```python
from build123d import *

# Parameters (mm, degrees)
EXTRUDE_1_DEPTH     = 4
SKETCH_3_R          = 9
EXTRUDE_2_DEPTH     = 7
SKETCH_4_R          = 3
CUT_EXTRUDE_1_DEPTH = 49.751330175
SKETCH_5_R          = 6
CUT_EXTRUDE_2_DEPTH = 10
SKETCH_7_R          = 5.5
CUT_EXTRUDE_3_DEPTH = 50.484262082
HOLE_WIZARD_M4_1_D  = 3.3
SCALE1_SCALE        = 2


with BuildPart() as part:
    # 草图1 → 凸台-拉伸1 (new body)
    with BuildSketch(Plane(origin=(0, 0, 0), x_dir=(1, 0, 0), z_dir=(0, 1, 0))):
        with BuildLine():
            Line((-8.109776452, 3.902758754), (-25.406517635, -32.039176982))
            ThreePointArc((-25.406517635, -32.039176982), (-23, -39.837168574), (-15.043482365, -38.022278184))
            Line((-15.043482365, -38.022278184), (0.302963304, -15.526261061))
            Line((0.302963304, -15.526261061), (7.351564548, -25.039059461))
            ThreePointArc((7.351564548, -25.039059461), (12.25592959, -26.282925824), (14.455537758, -21.72642235))
            Line((14.455537758, -21.72642235), (8.752682732, 2.095362733))
            ThreePointArc((8.752682732, 2.095362733), (0.95916746, 8.948742805), (-8.109776452, 3.902758754))
        make_face()
    extrude(amount=EXTRUDE_1_DEPTH)

    # 草图3 → 凸台-拉伸2 (add)
    with BuildSketch(Plane(origin=(0, 4, 0), x_dir=(1, 0, 0), z_dir=(0, 1, 0))):
        with Locations(Location((0, 0, 0), (0, 0, 154.301222305))):
            Circle(SKETCH_3_R)
    extrude(amount=EXTRUDE_2_DEPTH)

    # 草图4 → 切除-拉伸1 (cut, through all)
    with BuildSketch(Plane(origin=(0, 4, 0), x_dir=(1, 0, 0), z_dir=(0, 1, 0))):
        with Locations(Location((-20, -34.641016151, 0), (0, 0, 270))):
            Circle(SKETCH_4_R)
    extrude(amount=-CUT_EXTRUDE_1_DEPTH, mode=Mode.SUBTRACT)

    # 草图5 → 切除-拉伸2 (cut)
    with BuildSketch(Plane.XZ):
        with Locations(Location((0, 0, 0), (0, 0, 270))):
            Circle(SKETCH_5_R)
    extrude(amount=-CUT_EXTRUDE_2_DEPTH, mode=Mode.SUBTRACT)

    # 草图7 → 切除-拉伸3 (cut, through all)
    with BuildSketch(Plane(origin=(0, 11, 0), x_dir=(1, 0, 0), z_dir=(0, 1, 0))):
        with Locations(Location((0, 0, 0), (0, 0, 270))):
            Circle(SKETCH_7_R)
    extrude(amount=-CUT_EXTRUDE_3_DEPTH, mode=Mode.SUBTRACT)

    # M4 螺纹孔1 (through all)
    with Locations(Plane(origin=(0, 4, 0), x_dir=(1, 0, 0), z_dir=(0, 1, 0))):
        with Locations((10.565456544, -22.657694676)):
            Hole(HOLE_WIZARD_M4_1_D / 2)


with BuildPart() as part_1:
    # Scale1: scaled about (-4.168101576, 3.295275318, 12.285042226)
    add(part.part.scale(SCALE1_SCALE).moved(Location((4.168101576, -3.295275318, -12.285042226))))


solid = part_1.part
```
Design review of the part built by this model. Coordinates are the model's own, in mm. A direction names the side the tool comes from. Coordinates: 2 decimals unless noted, no trailing zeros. Order: outer loops, then holes, each group sorted by start corner. A loop starts at its lowest first (then second) coordinate and runs counter-clockwise, first axis right, second up. Notation, with made-up numbers: (68, -25) - (73, -25) arc R27 ccw to (73, 10) - close; hole circle Ø1 at (31, -23). An arc over 180 degrees is marked (long way). Answer in a Markdown table with one row per item.
(1) Clearance check with flat-ended pins moving along their axes: pin 1 (3 mm diameter, centred on y = 7, z = -1.5, fed in from -X); pin 2 (10.5 mm diameter, centred on x = 25.3, z = 33.03, fed in from +Y); pin 3 (2 mm diameter, centred on x = -1, y = 7, fed in from +Z). State where each tip first meets the part, or that it passes through.
Checked values:
| item | result |
|---|---|
| pin 1 | x = -11.25 |
| pin 2 | y = 4.7 |
| pin 3 | z = 5.23 |
(2) Consider section D-D on x = -39. State the section outline as (y, z) points.
Checked values:
| item | result |
|---|---|
| outline | (-3.3, 35.91) - (4.7, 35.91) - (4.7, 51.9) - (-3.3, 51.9) - close; (-3.3, 62.09) - (4.7, 62.09) - (4.7, 68.57) - (-3.3, 68.57) - close |
(3) Consider section B-B on y = 0. State the section outline as (x, z) points, plus the area to 3 significant figures.
Checked values:
| item | result |
|---|---|
| outline | (-46.64, 51.79) - (-12.05, -20.09) arc R18 ccw to (21.67, -16.48) - (33.08, 31.17) arc R8 ccw to (18.87, 37.79) - (4.77, 18.77) - (-25.92, 63.76) arc R12 ccw to start; hole circle Ø12 at (-35.83, 57); hole circle Ø24 at (4.17, -12.29); hole circle Ø6.6 at (25.3, 33.03) |
| area | 3,310 mm^2 |
(4) For faces 4 (the flat face through (-6, 16.705, -18)), 5 (the flat face through (-8, -3.295, 19)), 6 (the flat face through (-10.8, 0.6, 41.6)), list the 3-axis set-ups (+Z, -Z, +X, -X, +Y, -Y) from which the entire face can be reached by the end or side of a thin tool; tool diameter is ignored.
Checked values:
| item | result |
|---|---|
| face 4 | -Y |
| face 5 | +Z, -Z, +X, -X, -Y |
| face 6 | +Z, +Y, -Y |
(5) The part is to be moulded in two halves that separate along Z. For faces 1 (the flat face through (15, 18.705, -16)), 2 (the cylindrical face through (27.918, 0.649, 35.038)), 3 (the flat face through (-29.106, 0.649, 15.348)), say which applies: released by +Z, released by -Z, zero draft, split by the parting line, or undercut.
Checked values:
| item | result |
|---|---|
| face 1 | zero draft |
| face 2 | undercut |
| face 3 | released by -Z |
(6) Wall thickness on line 1 along Y through (x, z) = (-27.5, 17); line 2 along X through (y, z) = (14.25, -18); line 3 along Z through (x, y) = (10, 10.25): over which ranges is each line inside the solid? List them lowest first. Write a range as from..to.
Checked values:
| item | result |
|---|---|
| line 1 | -3.3..4.7 |
| line 2 | -12.9..-6.38, 14.72..21.24 |
| line 3 | -29.31..-22.77, -1.8..4.74 |
(7) Consider section C-C on z = -4. State the section outline as (x, y) points.
Checked values:
| item | result |
|---|---|
| outline | (-19.79, -3.3) - (-4.51, -3.3) - (-4.51, 16.7) - (-3.07, 16.7) - (-3.07, 18.7) - (-11.81, 18.7) - (-11.81, 4.7) - (-19.79, 4.7) - close; (11.4, 16.7) - (12.85, 16.7) - (12.85, -3.3) - (24.66, -3.3) - (24.66, 4.7) - (20.15, 4.7) - (20.15, 18.7) - (11.4, 18.7) - close |
(8) Consider section A-A on x = 9. State the section outline as (y, z) points.
Checked values:
| item | result |
|---|---|
| outline | (-3.3, -29.62) - (18.7, -29.62) - (18.7, -22.17) - (16.7, -22.17) - (16.7, -23.27) - (-3.3, -23.27) - close; (-3.3, -1.3) - (16.7, -1.3) - (16.7, -2.4) - (18.7, -2.4) - (18.7, 5.05) - (4.7, 5.05) - (4.7, 24.47) - (-3.3, 24.47) - close |
